Source: CAD feature listing. Evaluate the final solid. Frame: model axes, mm. Give positions to 0.01 mm unless a question says otherwise; leave off trailing zeros. Write each loop counter-clockwise with the first axis right and the second up, starting at its lowest first coordinate (ties: lowest second). Pieces come first, ordered by that corner, then holes. Notation, with made-up numbers: M 42.25,86.25 L 82.25,86.25 A6 cw 82.25,90.25 Z; hole C 70,68.25 d1. An arc over 180 degrees is marked long. Answer as a JSON object with one key per item and string values. Group by question number.
```python
from build123d import *

# Parameters (mm, degrees)
CROQUIS1_W              = 200
CROQUIS1_H              = 60
SALIENTE_EXTRUIR1_DEPTH = 1.55
REDONDEO1_R             = 15
CROQUIS2_R              = 7.5
CORTAR_EXTRUIR1_DEPTH   = 3.1


with BuildPart() as part:
    # Croquis1 → Saliente-Extruir1 (new body, symmetric)
    with BuildSketch(Plane(origin=(0, 0, 0), x_dir=(0, 0, -1), z_dir=(1, 0, 0))):
        Rectangle(CROQUIS1_W, CROQUIS1_H)
    extrude(amount=SALIENTE_EXTRUIR1_DEPTH, both=True)

    # Redondeo1
    redondeo1_edges = [part.edges().sort_by_distance(p)[0] for p in [
        (0, -30, -100),
        (0, -30, 100),
        (0, 30, 100),
        (0, 30, -100),
    ]]
    fillet(redondeo1_edges, radius=REDONDEO1_R)

    # Croquis2 → Cortar-Extruir1 (cut)
    with BuildSketch(Plane(origin=(1.55, 0, 0), x_dir=(0, 0, -1), z_dir=(1, 0, 0))):
        with Locations((-87.5, 0)):
            Circle(CROQUIS2_R)
        with Locations((87.5, 0)):
            Circle(CROQUIS2_R)
    extrude(amount=-CORTAR_EXTRUIR1_DEPTH, mode=Mode.SUBTRACT)


solid = part.part
```
(1) Pull-direction query (Z, two-part tool) for faces 1 (the cylindrical face through (0, 0, -80)), 2 (the cylindrical face through (0.02, -25.49, -95.72)), 3 (the flat face through (-1.55, 0, 1)), 4 (the cylindrical face through (0, 0, 95)); classes: pulls with the +Z half, pulls with the -Z half, needs draft (parallel to the pull), parting line crosses it, or undercut.
(2) Section A-A, the plane y = 0. Return loops of the section in (x, z).
(3) Section D-D, the plane y = 24.5. Return loops of the section in (x, z), plus the area to 3 significant figures.
(4) Section C-C, the plane z = -87.5. Return loops of the section in (x, y), plus the area to 3 significant figures.
(5) Ray query, L1, parallel to Y at x = -0.75, z = 87.5; L2, parallel to Y at x = -0.55, z = -85; L3, parallel to Z at x = 1.2, y = -6. Return the intervals inside material, ascending. Write a range as [from, to].
(6) Section B-B, the plane x = 0. Return loops of the section in (y, z).
Reported:
{
 "1": {"face 1": "undercut", "face 2": "pulls with the -Z half", "face 3": "needs draft", "face 4": "undercut"},
 "2": {"outline": "M -1.55,-100 L 1.55,-100 L 1.55,-95 L -1.55,-95 Z; M -1.55,-80 L 1.55,-80 L 1.55,80 L -1.55,80 Z; M -1.55,95 L 1.55,95 L 1.55,100 L -1.55,100 Z"},
 "3": {"outline": "M -1.55,-96.61 L 1.55,-96.61 L 1.55,96.61 L -1.55,96.61 Z", "area": "599 mm2"},
 "4": {"outline": "M -1.55,-29.79 L 1.55,-29.79 L 1.55,-7.5 L -1.55,-7.5 Z; M -1.55,7.5 L 1.55,7.5 L 1.55,29.79 L -1.55,29.79 Z", "area": "138 mm2"},
 "5": {"L1": "y = [-29.79, -7.5], [7.5, 29.79]", "L2": "y = [-30, -7.07], [7.07, 30]", "L3": "z = [-100, -92], [-83, 83], [92, 100]"},
 "6": {"outline": "M -30,-85 A15 ccw -15,-100 L 15,-100 A15 ccw 30,-85 L 30,85 A15 ccw 15,100 L -15,100 A15 ccw -30,85 Z; hole C 0,-87.5 d15; hole C 0,87.5 d15"}
}
